Model file for the job. Use its own axes, mm. A direction names the side the tool comes from. Coordinates: 2 decimals unless noted, no trailing zeros. Order: outer loops, then holes, each group sorted by start corner. A loop starts at its lowest first (then second) coordinate and runs counter-clockwise, first axis right, second up.
from build123d import *

# Parameters (mm, degrees)
SKETCH_1_R      = 1.5
EXTRUDE_1_DEPTH = 54


with BuildPart() as part:
    # 草图1 → 凸台-拉伸1 (new body)
    with BuildSketch(Plane.XY):
        with BuildLine():
            Line((-10.577234103, -3.535533906), (3.636038969, -3.535533906))
            ThreePointArc((3.636038969, -3.535533906), (4.401405834, -3.687774841), (5.050252532, -4.121320344))
            Line((5.050252532, -4.121320344), (5.525126266, -4.596194078))
            ThreePointArc((5.525126266, -4.596194078), (6.939339828, -5.181980515), (8.353553391, -4.596194078))
            Line((8.353553391, -4.596194078), (12.596194078, -0.353553391))
            ThreePointArc((12.596194078, -0.353553391), (13.181980515, 1.060660172), (12.596194078, 2.474873734))
            Line((12.596194078, 2.474873734), (12.121320344, 2.949747468))
            ThreePointArc((12.121320344, 2.949747468), (11.472473646, 3.383292971), (10.707106781, 3.535533906))
            Line((10.707106781, 3.535533906), (-1.535533906, 3.535533906))
            ThreePointArc((-1.535533906, 3.535533906), (-3.744957733, 3.782665284), (-5.845177969, 4.511844635))
            ThreePointArc((-5.845177969, 4.511844635), (-11.693982673, 3.369642712), (-12.295390172, -2.559223177))
            ThreePointArc((-12.295390172, -2.559223177), (-11.565318477, -3.27440977), (-10.577234103, -3.535533906))
        make_face()
        with Locations((-8, 0)):
            Circle(SKETCH_1_R, mode=Mode.SUBTRACT)
        with Locations((8, 0)):
            Circle(SKETCH_1_R, mode=Mode.SUBTRACT)
    extrude(amount=EXTRUDE_1_DEPTH)


solid = part.part
Q1. Cut at B-B, the plane z = 3.5. List the corners of the cut face in (x, y), plus the area to 3 significant figures.
Established:
outline: (-12.3, -2.56) arc R2 ccw to (-10.58, -3.54) - (3.64, -3.54) arc R2 cw to (5.05, -4.12) - (5.53, -4.6) arc R2 ccw to (8.35, -4.6) - (12.6, -0.35) arc R2 ccw to (12.6, 2.47) - (12.12, 2.95) arc R2 ccw to (10.71, 3.54) - (-1.54, 3.54) arc R10 cw to (-5.85, 4.51) arc R5 ccw to start; hole circle Ø3 at (-8, 0); hole circle Ø3 at (8, 0)
area: 172 mm2
Q2. Drop flat-ended pins along their axis: P1, Ø1.5, axis at x = 8, z = 42, coming from the -Y side; P2, Ø2, axis at y = -1.5, z = 16.5, coming from the +X side; P3, Ø11.5, axis at x = -4.5, z = 37, coming from the -Y side. Give the stop position or say it passes through.
Established:
P1: stops at y = -5.16
P2: stops at x = 12.45
P3: stops at y = -3.54
Q3. Cut at C-C, the plane x = 1. List the corners of the cut face in (y, z), plus the area to 3 significant figures.
Established:
outline: (-3.54, 0) - (3.54, 0) - (3.54, 54) - (-3.54, 54) - close
area: 382 mm2
Q4. Probe line 1 (X direction, y = -0.5, z = 49.5); line 2 (Y direction, x = -8, z = 39.5); line 3 (X direction, y = -1, z = 29.5). List the from-to ranges inside material, lowest first.
Established:
line 1: x = -12.97 to -9.41, -6.59 to 6.59, 9.41 to 12.45
line 2: y = -3.54 to -1.5, 1.5 to 5
line 3: x = -12.9 to -9.12, -6.88 to 6.88, 9.12 to 11.95
Q5. Mould opens along X. For faces 1 (the face through (10.45, -2.5, 26.62)), 2 (the face through (-9.5, 0.07, 26.62)), 3 (the face through (-12, 3, 27)), 4 (the face through (6.5, 0.07, 26.62)) say: pulls with the +X half, pulls with the -X half, needs draft (parallel to the pull), parting line crosses it, or undercut.
Established:
face 1: pulls with the +X half
face 2: undercut
face 3: parting line crosses it
face 4: undercut
Q6. Cut at A-A, the plane x = -8. List the corners of the cut face in (y, z), plus the area to 3 significant figures.
Established:
outline: (-3.54, 0) - (-1.5, 0) - (-1.5, 54) - (-3.54, 54) - close; (1.5, 0) - (5, 0) - (5, 54) - (1.5, 54) - close
area: 299 mm2
Q7. Which spindle directions (+Z, -Z, +X, -X, +Y, -Y) get a long thin tool onto all of the face, cutting with end or side? Do faces 5 (the face through (0, 0, 0)), 6 (the face through (5, 3.536, 27)), 7 (the face through (-4, -3.536, 27)). Say none if no direction does.
Established:
face 5: -Z, +X, -X, +Y, -Y
face 6: +Z, -Z, +X, +Y
face 7: +Z, -Z, -X, -Y
Q8. Cut at D-D, the plane x = -2.25. List the corners of the cut face in (y, z), plus the area to 3 significant figures.
Established:
outline: (-3.54, 0) - (3.56, 0) - (3.56, 54) - (-3.54, 54) - close
area: 383 mm2
